Read the model definition and answer for the solid it produces. Units are mm, in the model's axes. Face numbers are marked on the shaded views. A direction names the side the tool comes from. Give positions to 0.01 mm unless a question says otherwise; leave off trailing zeros. Loops run counter-clockwise (first coordinate to the right, second up) from the corner with the lowest first, then second, coordinate; pieces in that order, holes last.
(1) Find section B-B, the plane y = -4.75. Write down the section's boundary in (x, z) (3 decimals).
(2) Each of these flat-tipped pins is pushed along its axis until it touches: P1, Ø3, axis at x = 3, y = -7, coming from the +Z side; P2, Ø2.5, axis at x = -10, z = 7.5, coming from the -Y side; P3, Ø4, axis at y = -7, z = 8.5, coming from the -X side; P4, Ø1.6, axis at y = -5, z = 13, coming from the -X side. Where does it stop, or does it pass through?
(3) Find section D-D, the plane z = 10. Write down the section's boundary in (x, y), then the cut area to 3 significant figures.
(4) Which of the six approach directions +Z, -Z, +X, -X, +Y, -Y give full straight-line access (tool end or side, diameter ignored) to the marked faces 1, 2 and 3?
(5) Find section C-C, the plane x = 1.25. Write down the section's boundary in (y, z), then the cut area to 3 significant figures.
(6) Find section A-A, the plane z = 5. Write down the section's boundary in (x, y).
(7) Straight lines are drawn through the part: probe 1 along Y at (x, z) = (-8.25, 11.25); probe 2 along X at (y, z) = (-4.75, 14); probe 3 along X at (y, z) = (-3, 9). For each, find the intervals that lie inside material, in ascending order.
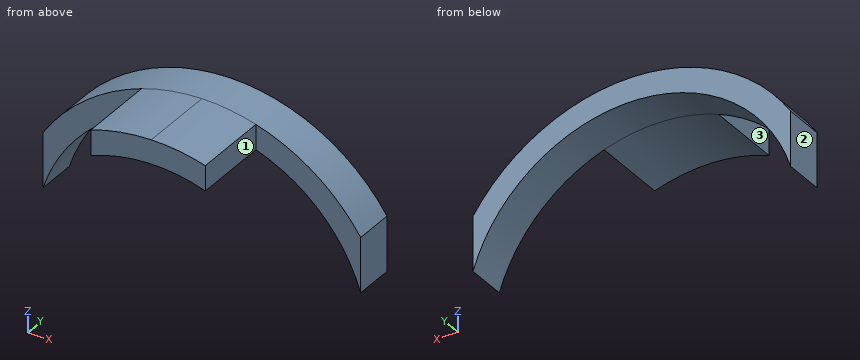
```python
from build123d import *

# Parameters (mm, degrees)
F1_DEPTH = 3.302
F3_DEPTH = 6.35


with BuildPart() as f1:
    # F0 (on Front) → F1 (new body)
    with BuildSketch(Plane.XZ):
        with BuildLine():
            Line((12.7, 4.0659838908), (12.7, 8.4242269675))
            ThreePointArc((12.7, 8.4242269675), (0, 15.24), (-12.7, 8.4242269675))
            Line((-12.7, 8.4242269675), (-12.7, 4.0659838908))
            ThreePointArc((-12.7, 4.0659838908), (0, 13.335), (12.7, 4.0659838908))
        make_face()
    extrude(amount=F1_DEPTH)

    # F2 (on face) → F3 (join)
    with BuildSketch(Plane.XZ.offset(3.302)):
        with BuildLine():
            ThreePointArc((4.3219749297, 14.6143125978), (2.1835150571, 15.0827670537), (0, 15.24))
            ThreePointArc((0, 15.24), (-2.4425893067, 15.0429836628), (-4.8220250703, 14.4570285405))
            Line((-4.8220250703, 14.4570285405), (-4.8220250703, 12.4326304225))
            ThreePointArc((-4.8220250703, 12.4326304225), (-0.2661645943, 13.3323434327), (4.3219749297, 12.6151796542))
            Line((4.3219749297, 12.6151796542), (4.3219749297, 14.6143125978))
        make_face()
    extrude(amount=F3_DEPTH)


solid = f1.part
```
Entries:
1. outline: (-4.822, 12.433) arc R13.335 cw to (4.322, 12.615) - (4.322, 14.614) arc R15.24 ccw to (-4.822, 14.457) - close
2. P1: stops at z = 15.17
2. P2: stops at y = -3.3
2. P3: passes through
2. P4: stops at x = -4.82
3. outline: (-11.5, -3.3) - (-8.82, -3.3) - (-8.82, 0) - (-11.5, 0) - close; (8.82, -3.3) - (11.5, -3.3) - (11.5, 0) - (8.82, 0) - close
3. area: 17.7 mm2
4. face 1: +Z, -Z, +X, -Y
4. face 2: +Z, -Z, -X, +Y, -Y
4. face 3: +Z, -Z, -X, -Y
5. outline: (-9.65, 13.28) - (0, 13.28) - (0, 15.19) - (-9.65, 15.19) - close
5. area: 18.5 mm2
6. outline: (-12.7, -3.3) - (-12.36, -3.3) - (-12.36, 0) - (-12.7, 0) - close; (12.36, -3.3) - (12.7, -3.3) - (12.7, 0) - (12.36, 0) - close
7. probe 1: y = -3.3 to 0
7. probe 2: x = -4.82 to 4.32
7. probe 3: x = -12.3 to -9.84, 9.84 to 12.3
